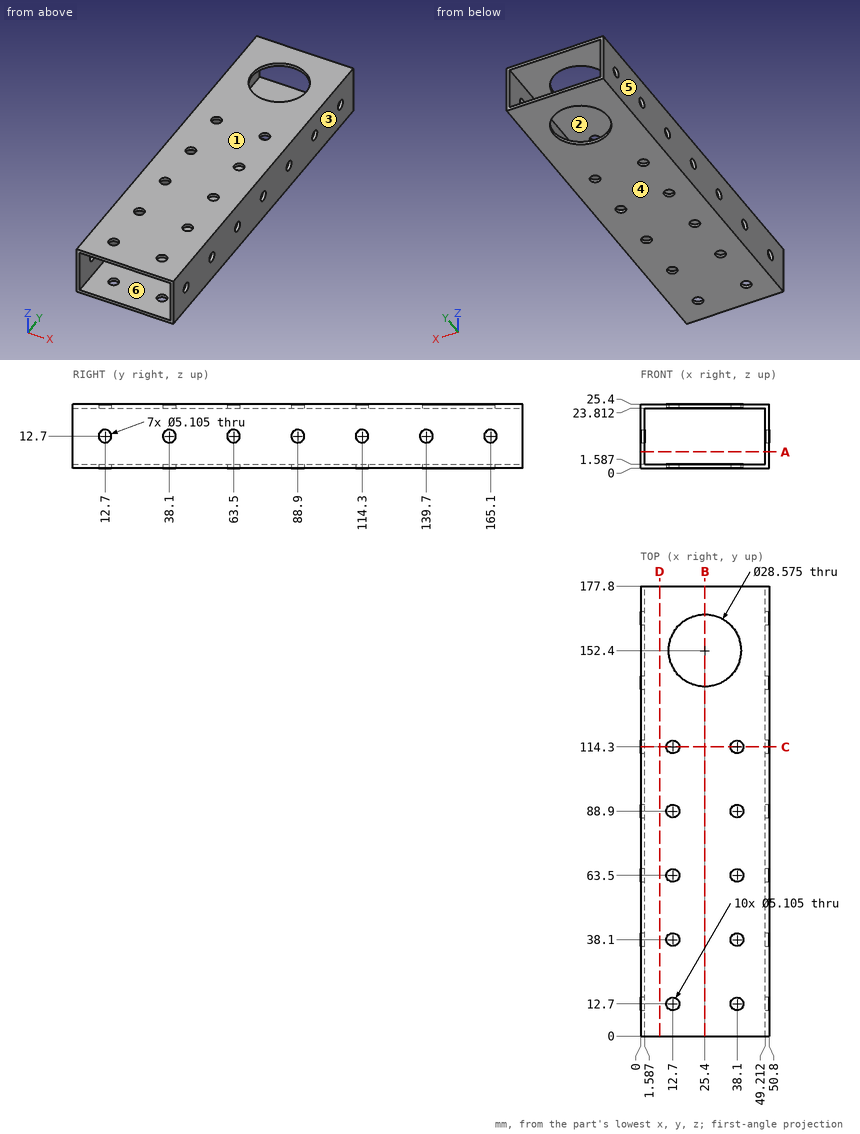
Answer from the drawing. Dimensions are ordinates in mm from the lowest x, y and z of the part. A direction names the side the tool comes from. Round coordinates to 2 decimals unless told otherwise and drop trailing zeros. Loops run counter-clockwise (first coordinate to the right, second up) from the corner with the lowest first, then second, coordinate; pieces in that order, holes last.
Q1. Consider probe 1 along Z at (x, y) = (32, 31.5); probe 2 along X at (y, z) = (43.5, 16.5); probe 3 along Z at (x, y) = (49.85, 38.1). Determine where each line is inside the solid, lowest interval first.
Q2. This flat-tipped pin is pushed along its axis until it touches: pin 1 (4 mm diameter, centred on y = 165.1, z = 12.7, fed in from -X). Where does it stop, or does it pass through?
Q3. Section A-A on z = 6.5 is taken. Write down the section's boundary in (x, y).
Q4. Section B-B on x = 25.4 is taken. Write down the section's boundary in (y, z).
Q5. Section C-C on y = 114.3 is taken. Give the number of separate pieces and of enclosed holes in the cut face, and give its area (3 significant figures).
Q6. Determine the mould class of the marked faces 3, 4, 5 and 6 for opening direction X: released by +X, released by -X, zero draft, split by the parting line, or undercut.
Q7. Which of the six approach directions +Z, -Z, +X, -X, +Y, -Y give full straight-line access (tool end or side, diameter ignored) to the marked faces 1 and 2?
Q8. Section D-D on x = 7.5 is taken. Write down the section's boundary in (y, z).
Output:
1. probe 1: z = 0 to 1.59, 23.81 to 25.4
1. probe 2: x = 0 to 1.59, 49.21 to 50.8
1. probe 3: z = 0 to 10.15, 15.25 to 25.4
2. pin 1: passes through
3. outline: (0, 0) - (1.59, 0) - (1.59, 177.8) - (0, 177.8) - close; (49.21, 0) - (50.8, 0) - (50.8, 177.8) - (49.21, 177.8) - close
4. outline: (0, 0) - (138.11, 0) - (138.11, 1.59) - (0, 1.59) - close; (0, 23.81) - (138.11, 23.81) - (138.11, 25.4) - (0, 25.4) - close; (166.69, 0) - (177.8, 0) - (177.8, 1.59) - (166.69, 1.59) - close; (166.69, 23.81) - (177.8, 23.81) - (177.8, 25.4) - (166.69, 25.4) - close
5. separate pieces: 6
5. enclosed holes: 0
5. area: 183 mm2
6. face 3: released by +X
6. face 4: zero draft
6. face 5: released by -X
6. face 6: undercut
7. face 1: +Z, +X, -X, +Y, -Y
7. face 2: +Y, -Y
8. outline: (0, 0) - (177.8, 0) - (177.8, 1.59) - (0, 1.59) - close; (0, 23.81) - (177.8, 23.81) - (177.8, 25.4) - (0, 25.4) - close
